from build123d import *

# Parameters (mm, degrees)
SKETCH3_R           = 10
BOSS_EXTRUDE2_DEPTH = 50
SKETCH3_4_R         = 10
BOSS_EXTRUDE3_DEPTH = 15
CHAMFER1_SIZE       = 50
CHAMFER1_SIZE2      = 25


with BuildPart() as part:
    # Sketch3 → Boss-Extrude2 (new body)
    with BuildSketch(Plane.XY):
        with BuildLine():
            Line((90, -7.5), (90, 7.5))
            Line((90, 7.5), (18.540496218, 7.5))
            ThreePointArc((18.540496218, 7.5), (15.215049384, 12.980842508), (10.326323506, 17.127960849))
            ThreePointArc((10.326323506, 17.127960849), (-18.972544219, -6.327919552), (18.540496218, -7.5))
            Line((18.540496218, -7.5), (90, -7.5))
        make_face()
        Circle(SKETCH3_R, mode=Mode.SUBTRACT)
    extrude(amount=BOSS_EXTRUDE2_DEPTH)

    # Sketch3<4> → Boss-Extrude3 (add)
    with BuildSketch(Plane.XY):
        with BuildLine():
            Line((90, 7.5), (90, 25))
            ThreePointArc((90, 25), (73.405373459, 44.707953511), (51.15965684, 31.711294182))
            ThreePointArc((51.15965684, 31.711294182), (34.200595531, 14.738332513), (10.326323506, 17.127960849))
            ThreePointArc((10.326323506, 17.127960849), (15.215049384, 12.980842508), (18.540496218, 7.5))
            Line((18.540496218, 7.5), (90, 7.5))
        make_face()
        with Locations((70, 25)):
            Circle(SKETCH3_4_R, mode=Mode.SUBTRACT)
    extrude(amount=BOSS_EXTRUDE3_DEPTH)

    # Chamfer1
    chamfer1_edges = [part.edges().sort_by_distance(p)[0] for p in [
        (90, 0, 50),
    ]]
    chamfer1_side = [part.faces().sort_by_distance(p)[0] for p in [
        (28.950156373, 0, 50),
    ]]
    chamfer(chamfer1_edges, length=CHAMFER1_SIZE, length2=CHAMFER1_SIZE2, reference=chamfer1_side[0])


solid = part.part
Check sheet for the modelled part. Datum: model origin and axes. Units: mm. A direction names the side the tool comes from. Give positions to 0.01 mm unless a question says otherwise; leave off trailing zeros. Loops run counter-clockwise (first coordinate to the right, second up) from the corner with the lowest first, then second, coordinate; pieces in that order, holes last. Notation, with made-up numbers: M 30,44.5 L 87,44.5 A10 cw 87,51.5 Z; hole C -16.75,61 d4. An arc over 180 degrees is marked long. Return JSON: item names as keys, results as strings. Group by question number.
1. Go/stop test with flat-tipped pins: pin 1 (2 mm diameter, centred on x = 48, y = 24.5, fed in from +Z); pin 2 (4 mm diameter, centred on y = -6, z = 19, fed in from -X); pin 3 (12 mm diameter, centred on y = -8.5, z = 42.5, fed in from +X). Record where each tip stops, or that it passes through.
2. Tool access check on faces 5 (the flat face through (65.4, -0.1, 37.3)), 6 (the flat face through (58, 22, 15)). Record the directions out of +Z, -Z, +X, -X, +Y, -Y that give a thin tool (end or side, any length) a straight path to the whole face; none if there is none.
3. Cross-section at C-C on z = 29.5. Record the boundary of the cut face in (x, y), plus the area to 3 significant figures.
4. Cross-section at B-B on x = 70. Record the boundary of the cut face in (y, z), plus the area to 4 significant figures.
5. Thickness scan on L1, parallel to Y at x = 0, z = 18; L2, parallel to Y at x = 70, z = 7; L3, parallel to Y at x = 45.5, z = 41. Record the ranges inside material, lowest first.
6. Mould release check, pull along Y, two halves, no side actions. Record for faces 1 (the cylindrical face through (60, 25, 7)), 2 (the cylindrical face through (-2.17, -9.76, 24.65)), 3 (the flat face through (54, -7.5, 19)), 4 (the flat face through (10, -4, 50)): released by +Y, released by -Y, zero draft, split by the parting line, or undercut.
7. Cross-section at A-A on y = 0. Record the boundary of the cut face in (x, z), plus the area to 4 significant figures.
8. Cross-section at D-D on x = 0. Record the boundary of the cut face in (y, z).
Return value:
{
 "1": {"pin 1": "z = 15", "pin 2": "x = -19.6", "pin 3": "x = 66.83"},
 "2": {"face 5": "+Z, +X, +Y, -Y", "face 6": "+Z, +X, +Y"},
 "3": {"outline": "M 18.54,-7.5 L 81,-7.5 L 81,7.5 L 18.54,7.5 A20 ccw long Z; hole C 0,0 d20", "area": "1,860 mm^2"},
 "4": {"outline": "M -7.5,0 L 15,0 L 15,15 L 7.5,15 L 7.5,35 L -7.5,35 Z; M 35,0 L 45,0 L 45,15 L 35,15 Z", "area": "787.5 mm^2"},
 "5": {"L1": "-20 to -10, 10 to 20", "L2": "-7.5 to 15, 35 to 45", "L3": "-7.5 to 7.5"},
 "6": {"face 1": "undercut", "face 2": "undercut", "face 3": "released by -Y", "face 4": "zero draft"},
 "7": {"outline": "M -20,0 L -10,0 L -10,50 L -20,50 Z; M 10,0 L 90,0 L 90,25 L 40,50 L 10,50 Z", "area": "3,875 mm^2"},
 "8": {"outline": "M -20,0 L -10,0 L -10,50 L -20,50 Z; M 10,0 L 20,0 L 20,50 L 10,50 Z"}
}
